Input: part model. Units: mm. Frame: model coordinates. Give positions to 0.01 mm unless a question says otherwise; leave off trailing zeros. Write each loop counter-clockwise with the first axis right and the second up, starting at its lowest first coordinate (ties: lowest second). Pieces come first, ordered by that corner, then holes. Notation, with made-up numbers: (31, -28.5) - (81, -28.5) arc R32 cw to (81, -0.5) - close; hole circle Ø8 at (-24, -12). An arc over 180 degrees is marked (long way). Answer as a JSON object with one key per item and string values. Group by question number.
Autodesk Inventor part; units mm, degrees
ref_plane "Work Plane1" through (-24.15, -24.15, 49.8) normal (0, 0, 1) x (1, 0, 0)
ref_plane "YZ Plane" through (0, 0, 0) normal (1, 0, 0) x (0, 1, 0)
ref_plane "XZ Plane" through (0, 0, 0) normal (0, 1, 0) x (-1, 0, 0)
sketch "Sketch1" plane through (0, 0, 0) normal (0, 0, 1) x (1, 0, 0)
  circle A0 centre (-21.9, -21.9) radius 1.875
  circle A1 centre (21.9, 21.9) radius 1.875
  circle A2 centre (21.9, -21.9) radius 1.875
  circle A3 centre (-21.9, 21.9) radius 1.875
  circle A4 centre (14.4, 20.8) radius 2.0675
  circle A5 centre (-14.4, -20.8) radius 2.0675
  circle A6 centre (14.4, -20.8) radius 2.0675
  circle A7 centre (20.8, -14.4) radius 2.0675
  line L0 (-17.05, 17.05) -> (-17.05, -17.05)
  line L1 (17.05, 17.05) -> (-17.05, 17.05)
  line L2 (17.05, -17.05) -> (17.05, 17.05)
  line L3 (-17.05, -17.05) -> (17.05, -17.05)
  circle A8 centre (20.8, 14.4) radius 2.0675
  circle A9 centre (-14.4, 20.8) radius 2.0675
  circle A10 centre (-20.8, -14.4) radius 2.0675
  circle A11 centre (-20.8, 14.4) radius 2.0675
  line L4 (-22.9, 24.15) -> (22.9, 24.15)
  arc A12 (-22.9, 24.15) -> (-24.15, 22.9) centre (-22.9, 22.9) ccw
  line L5 (-24.15, -22.9) -> (-24.15, 22.9)
  arc A13 (-24.15, -22.9) -> (-22.9, -24.15) centre (-22.9, -22.9) ccw
  line L6 (22.9, -24.15) -> (-22.9, -24.15)
  arc A14 (22.9, -24.15) -> (24.15, -22.9) centre (22.9, -22.9) ccw
  line L7 (24.15, 22.9) -> (24.15, -22.9)
  arc A15 (24.15, 22.9) -> (22.9, 24.15) centre (22.9, 22.9) ccw
  point P0 (0, 0)
ref_plane "Work Plane1" through (-24.15, -24.15, 49.8) normal (0, 0, 1) x (1, 0, 0)
extrude "Extrusion1" add sketch "Sketch1" along normal blind 1.5 from surface at 49.8 contours A0 | A1 | A2 | A3 | L1 L2 L3 L0 | L4 A15 L7 A14 L6 A13 L5 A12
sketch "Sketch2" plane through (-22.9, -24.15, 51.3) normal (0, 0, 1) x (1, 0, 0)
  arc A0 (-1.25, 1.25) -> (0, 0) centre (0, 1.25) ccw
  line L0 (45.8, 0) -> (0, 0)
  arc A1 (45.8, 0) -> (47.05, 1.25) centre (45.8, 1.25) ccw
  line L1 (47.05, 47.05) -> (47.05, 1.25)
  arc A2 (47.05, 47.05) -> (45.8, 48.3) centre (45.8, 47.05) ccw
  line L2 (0, 48.3) -> (45.8, 48.3)
  arc A3 (0, 48.3) -> (-1.25, 47.05) centre (0, 47.05) ccw
  line L3 (-1.25, 1.25) -> (-1.25, 47.05)
  circle A4 centre (2.1, 38.55) radius 2.0675
  circle A5 centre (2.1, 9.75) radius 2.0675
  circle A6 centre (8.5, 44.95) radius 2.0675
  circle A7 centre (43.7, 38.55) radius 2.0675
  circle A8 centre (43.7, 9.75) radius 2.0675
  circle A9 centre (37.3, 3.35) radius 2.0675
  circle A10 centre (8.5, 3.35) radius 2.0675
  circle A11 centre (37.3, 44.95) radius 2.0675
  arc A12 (47.9, 47.05) -> (45.8, 49.15) centre (45.8, 47.05) ccw
  line L4 (47.9, 47.05) -> (47.9, 1.25)
  arc A13 (45.8, -0.85) -> (47.9, 1.25) centre (45.8, 1.25) ccw
  line L5 (45.8, -0.85) -> (0, -0.85)
  arc A14 (-2.1, 1.25) -> (0, -0.85) centre (0, 1.25) ccw
  line L6 (-2.1, 1.25) -> (-2.1, 47.05)
  arc A15 (0, 49.15) -> (-2.1, 47.05) centre (0, 47.05) ccw
  line L7 (0, 49.15) -> (45.8, 49.15)
  line L8 (47.05, 1.25) -> (45.8, 1.25)
  line L9 (45.8, 1.25) -> (45.8, -0.85)
  line L10 (45.8, -0.85) -> (47.05, -0.85)
  line L11 (47.05, -0.85) -> (47.05, 1.25)
  line L12 (-1.25, 1.25) -> (0, 1.25)
  line L13 (0, 1.25) -> (0, -0.85)
  line L14 (0, -0.85) -> (-1.25, -0.85)
  line L15 (-1.25, -0.85) -> (-1.25, 1.25)
  line L16 (-1.25, 47.05) -> (0, 47.05)
  line L17 (0, 47.05) -> (0, 49.15)
  line L18 (0, 49.15) -> (-1.25, 49.15)
  line L19 (-1.25, 49.15) -> (-1.25, 47.05)
  line L20 (47.05, 47.05) -> (45.8, 47.05)
  line L21 (45.8, 47.05) -> (45.8, 49.15)
  line L22 (45.8, 49.15) -> (47.05, 49.15)
  line L23 (47.05, 49.15) -> (47.05, 47.05)
  point P0 (22.9, 24.15)
  dimension "d2" = 0.85
extrude "Extrusion2" add sketch "Sketch2" against normal blind 1.5 contours A0 L13 A14 L15 | L0 L9 L5 L13 | L19 A15 L17 A3 | A14 L14 L15 | A1 L11 A13 L9 | L17 L7 L21 L2 | L19 L18 A15 | A13 L11 L10 | L21 A12 L23 A2 | L22 L23 A12
pattern_linear "Rectangular Pattern1" count 3 spacing 50 along (0, 1, 0) of "Extrusion1", "Extrusion2"
chamfer "Chamfer1" distance 1.5 angle 45 2 edges at (0, -25, 51.3) (0, 125, 51.3)
properties part number "Panel Top 1x3"
1) Cut plane A-A on x = 14.4. Count the separate pieces of the cut face and the enclosed holes in it, and give its area (3 significant figures).
2) Line query: line 1 along X through (y, z) = (19.5, 50); line 2 along X through (y, z) = (64, 50.45); line 3 along Y through (x, z) = (-2, 51.25). Output: solid intervals per line, ascending. Write a range as from..to.
3) Mould query, pull axis X, two halves, no side actions, for faces 1 (the face through (-14.67, 27.15, 50.54)), 2 (the face through (21.911, 62.657, 50.54)), 3 (the face through (0, 51, 51.3)). Classes: +X half, -X half, draft (parallel to the pull), parting line (faces both ways), or undercut.
4) Cut plane B-B on y = 120.8. Return the cut outline in (x, z).
5) Pin query (flat end, axial travel): P1, Ø3.5, axis at x = 20.8, y = 85.6, coming from the +Z side. Return the tip coordinate at first contact, or that it passes through.
Filled in:
{
 "1": {"separate pieces": "7", "enclosed holes": "0", "area": "186 mm²"},
 "2": {"line 1": "x = -24.15..-16.01, -12.79..12.79, 16.01..24.15", "line 2": "x = -24.15..-22.83, -18.77..18.77, 22.83..24.15", "line 3": "y = -23.55..123.55"},
 "3": {"face 1": "undercut", "face 2": "undercut", "face 3": "draft"},
 "4": {"outline": "(-24.15, 49.8) - (-16.47, 49.8) - (-16.47, 51.3) - (-24.15, 51.3) - close; (-12.33, 49.8) - (12.33, 49.8) - (12.33, 51.3) - (-12.33, 51.3) - close; (16.47, 49.8) - (24.15, 49.8) - (24.15, 51.3) - (16.47, 51.3) - close"},
 "5": {"P1": "passes through"}
}
